Source: CAD feature listing. Evaluate the final solid. Frame: model axes, mm. Give positions to 0.01 mm unless a question says otherwise; leave off trailing zeros. Order: outer loops, then holes, each group sorted by start corner. A loop starts at its lowest first (then second) coordinate and runs counter-clockwise, first axis right, second up.
1) Section A-A, the plane x = 43. Return loops of the section in (y, z).
2) Material intervals for line 1 (Y direction, x = 22.5, z = 1); line 2 (Y direction, x = -103, z = 0.5); line 3 (X direction, y = -12.5, z = 1.9), sorted ascending.
3) Section B-B, the plane x = 23.5. Return loops of the section in (y, z).
4) Section C-C, the plane y = -31. Return loops of the section in (x, z), plus the area to 3 significant figures.
5) Section D-D, the plane z = 0.6. Return loops of the section in (x, y).
6) First-contact query: P1, Ø1.2, axis at x = -120, z = 1, coming from the +Y side; P2, Ø1.2, axis at y = 29, z = 1, coming from the -X side; P3, Ø4.5, axis at x = -104.18, y = -24.01, coming from the +Z side; P4, Ø0.7, axis at y = -33, z = 1, coming from the +X side. Flat tips, straight axial feed; report the tip coordinate or a pass-through.
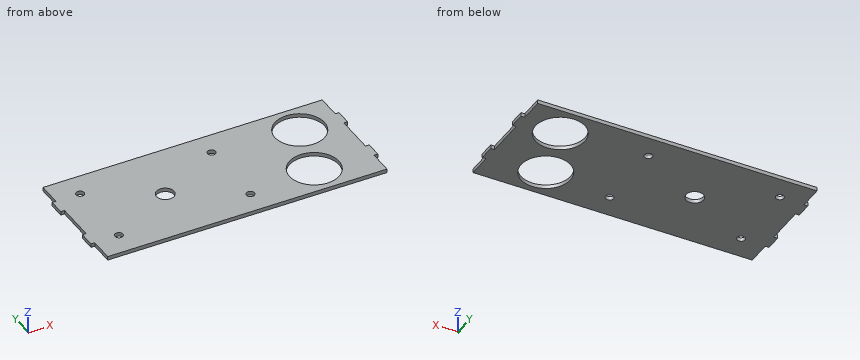
```python
from build123d import *

# Parameters (mm, degrees)
BOSS_EXTRUDE1_DEPTH = 2.3622
SKETCH2_R           = 15.5
SKETCH2_R_2         = 5.5
SKETCH2_R_3         = 2.5
CUT_EXTRUDE1_DEPTH  = 128.843896579


with BuildPart() as part:
    # Sketch1 → Boss-Extrude1 (new body)
    with BuildSketch(Plane.XY):
        Polygon((-119.363142231, 35.994577783), (-119.363142231, 20.994577783), (-121.725342231, 20.994577783), (-121.725342231, 10.994577783), (-119.363142231, 10.994577783), (-119.363142231, -14.005422217), (-121.725342231, -14.005422217), (-121.725342231, -24.005422217), (-119.363142231, -24.005422217), (-119.363142231, -39.005422217), (55.912457769, -39.005422217), (55.912457769, -24.005422217), (58.274657769, -24.005422217), (58.274657769, -14.005422217), (55.912457769, -14.005422217), (55.912457769, 10.994577783), (58.274657769, 10.994577783), (58.274657769, 20.994577783), (55.912457769, 20.994577783), (55.912457769, 35.994577783), align=None)
    extrude(amount=BOSS_EXTRUDE1_DEPTH)

    # Sketch2 → Cut-Extrude1 (cut, through all)
    with BuildSketch(Plane.XY.offset(2.3622)):
        with Locations((31.328134445, 16.721516998)):
            Circle(SKETCH2_R)
        with Locations((20.753669958, -19.61125842)):
            Circle(SKETCH2_R)
        with Locations((-62.931965905, -1.505422217)):
            Circle(SKETCH2_R_2)
        with Locations((-104.181965905, 20.994577783)):
            Circle(SKETCH2_R_3)
        with Locations((-21.681965905, 20.994577783)):
            Circle(SKETCH2_R_3)
        with Locations((-21.681965905, -24.005422217)):
            Circle(SKETCH2_R_3)
        with Locations((-104.181965905, -24.005422217)):
            Circle(SKETCH2_R_3)
    extrude(amount=-CUT_EXTRUDE1_DEPTH, mode=Mode.SUBTRACT)


solid = part.part
```
From the geometry:
1. outline: (-39.01, 0) - (6.52, 0) - (6.52, 2.36) - (-39.01, 2.36) - close; (26.92, 0) - (35.99, 0) - (35.99, 2.36) - (26.92, 2.36) - close
2. line 1: y = -39.01 to -35.01, -4.21 to 3.98, 29.46 to 35.99
2. line 2: y = -39.01 to -26.21, -21.8 to 18.79, 23.2 to 35.99
2. line 3: x = -119.36 to 6.98, 34.53 to 55.91
3. outline: (-39.01, 0) - (-34.87, 0) - (-34.87, 2.36) - (-39.01, 2.36) - close; (-4.36, 0) - (3.34, 0) - (3.34, 2.36) - (-4.36, 2.36) - close; (30.1, 0) - (35.99, 0) - (35.99, 2.36) - (30.1, 2.36) - close
4. outline: (-119.36, 0) - (10.24, 0) - (10.24, 2.36) - (-119.36, 2.36) - close; (31.27, 0) - (55.91, 0) - (55.91, 2.36) - (31.27, 2.36) - close
4. area: 364 mm2
5. outline: (-121.73, -24.01) - (-119.36, -24.01) - (-119.36, -39.01) - (55.91, -39.01) - (55.91, -24.01) - (58.27, -24.01) - (58.27, -14.01) - (55.91, -14.01) - (55.91, 10.99) - (58.27, 10.99) - (58.27, 20.99) - (55.91, 20.99) - (55.91, 35.99) - (-119.36, 35.99) - (-119.36, 20.99) - (-121.73, 20.99) - (-121.73, 10.99) - (-119.36, 10.99) - (-119.36, -14.01) - (-121.73, -14.01) - close; hole circle Ø5 at (-104.18, -24.01); hole circle Ø5 at (-104.18, 20.99); hole circle Ø11 at (-62.93, -1.51); hole circle Ø5 at (-21.68, -24.01); hole circle Ø5 at (-21.68, 20.99); hole circle Ø31 at (20.75, -19.61); hole circle Ø31 at (31.33, 16.72)
6. P1: stops at y = 20.99
6. P2: stops at x = -119.36
6. P3: passes through
6. P4: stops at x = 55.91
